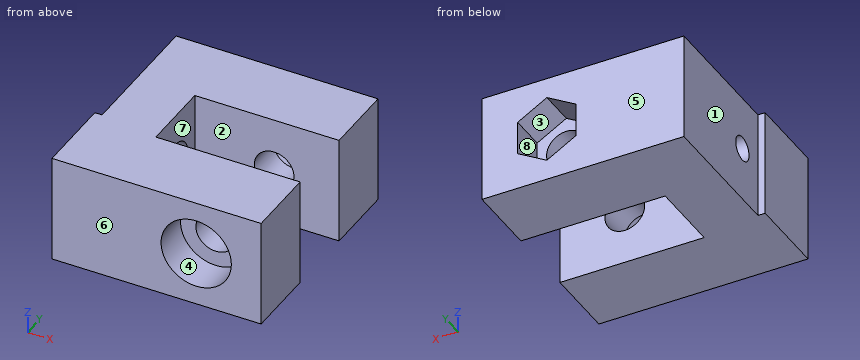
```python
from build123d import *

# Parameters (mm, degrees)
F1_DEPTH       = 15
F3_D           = 5.5
F3_CBORE_D     = 9.75
F3_CBORE_DEPTH = 5
F5_D           = 3.4
F5_CBORE_D     = 6.5
F5_CBORE_DEPTH = 3
F7_DEPTH       = 5


with BuildPart() as f1:
    # F0 (on Top) → F1 (new body)
    with BuildSketch(Plane.XY):
        Polygon((0, 15), (0, 0), (0, -4), (-1, -4), (-1, -15), (28, -15), (28, -5), (8, -5), (8, 0), (8, 5), (28, 5), (28, 15), align=None)
    extrude(amount=F1_DEPTH)

    # F3 (through all)
    with Locations(Plane.XZ.offset(15)):
        with Locations((19, 7.5)):
            CounterBoreHole(F3_D / 2, F3_CBORE_D / 2, F3_CBORE_DEPTH)

    # F5 (through all)
    with Locations(Plane.YZ.offset(8)):
        with Locations((0, 7.5)):
            CounterBoreHole(F5_D / 2, F5_CBORE_D / 2, F5_CBORE_DEPTH)

    # F6 (on face) → F7 (cut)
    with BuildSketch(Plane(origin=(0, 15, 0), x_dir=(-1, 0, 0), z_dir=(0, 1, 0))):
        Polygon((-23.05, 5.1617314098), (-19, 2.8234628196), (-14.95, 5.1617314098), (-14.95, 9.8382685902), (-19, 12.1765371804), (-23.05, 9.8382685902), align=None)
    extrude(amount=-F7_DEPTH, mode=Mode.SUBTRACT)


solid = f1.part
```
Verification items for the finished model (mm, model axes). Face numbers are marked on the shaded views. A direction names the side the tool comes from. Round coordinates to 2 decimals unless told otherwise and drop trailing zeros. Write each loop counter-clockwise with the first axis right and the second up, starting at its lowest first coordinate (ties: lowest second). Pieces come first, ordered by that corner, then holes.
1. Scan lines: L1, parallel to Y at x = 21, z = 3.5; L2, parallel to Y at x = 21.75, z = 8.5; L3, parallel to Z at x = 19, y = -12.35 (3 decimals). Record each from-to range of solid material in increasing order.
2. Section check C-C on x = 11.5. Enter the section's corners in (y, z).
3. Draft check along Y on the marked faces 6, 7 and 8. Enter one of: +Y half, -Y half, draft (parallel to the pull), parting line (faces both ways), or undercut.
4. Section check A-A on z = 7.5. State how many separate pieces and enclosed holes the cut face has, plus the area to 3 significant figures.
5. Gauge pin test, flat ends, axial feed: P1, Ø6.5, axis at x = 17, z = 7.5, coming from the +Y side; P2, Ø5.5, axis at y = 0, z = 7.5, coming from the +X side; P3, Ø5, axis at y = 0, z = 7.5, coming from the -X side; P4, Ø6, axis at x = 19, z = 7.5, coming from the -Y side. Record the tip position at first contact, or that the pin passes through.
6. Section check D-D on y = 0. Enter the section's corners in (x, z).
7. Section check B-B on y = 11. Enter the section's corners in (x, z).
8. Access from +Z, -Z, +X, -X, +Y, -Y to the whole of each face (thin tool, end or side, straight path). Record for the marked faces 1, 2, 3, 4 and 5.
Answer:
1. L1: y = -10 to -5, 5 to 15
1. L2: y = -10 to -5, 5 to 10
1. L3: z = 0 to 2.625, 12.375 to 15
2. outline: (-15, 0) - (-5, 0) - (-5, 15) - (-15, 15) - close; (5, 0) - (15, 0) - (15, 15) - (5, 15) - close
3. face 6: -Y half
3. face 7: undercut
3. face 8: draft
4. separate pieces: 4
4. enclosed holes: 0
4. area: 470 mm2
5. P1: stops at y = 15
5. P2: stops at x = 5
5. P3: stops at x = 0
5. P4: stops at y = -10
6. outline: (0, 0) - (8, 0) - (8, 4.25) - (5, 4.25) - (5, 5.8) - (0, 5.8) - close; (0, 9.2) - (5, 9.2) - (5, 10.75) - (8, 10.75) - (8, 15) - (0, 15) - close
7. outline: (0, 0) - (28, 0) - (28, 15) - (0, 15) - close; hole (14.95, 5.16) - (19, 2.82) - (23.05, 5.16) - (23.05, 9.84) - (19, 12.18) - (14.95, 9.84) - close
8. face 1: +Z, -Z, -X, +Y
8. face 2: +Z, -Z, +X
8. face 3: +Y
8. face 4: -Y
8. face 5: +Z, -Z, +X, -X, +Y
